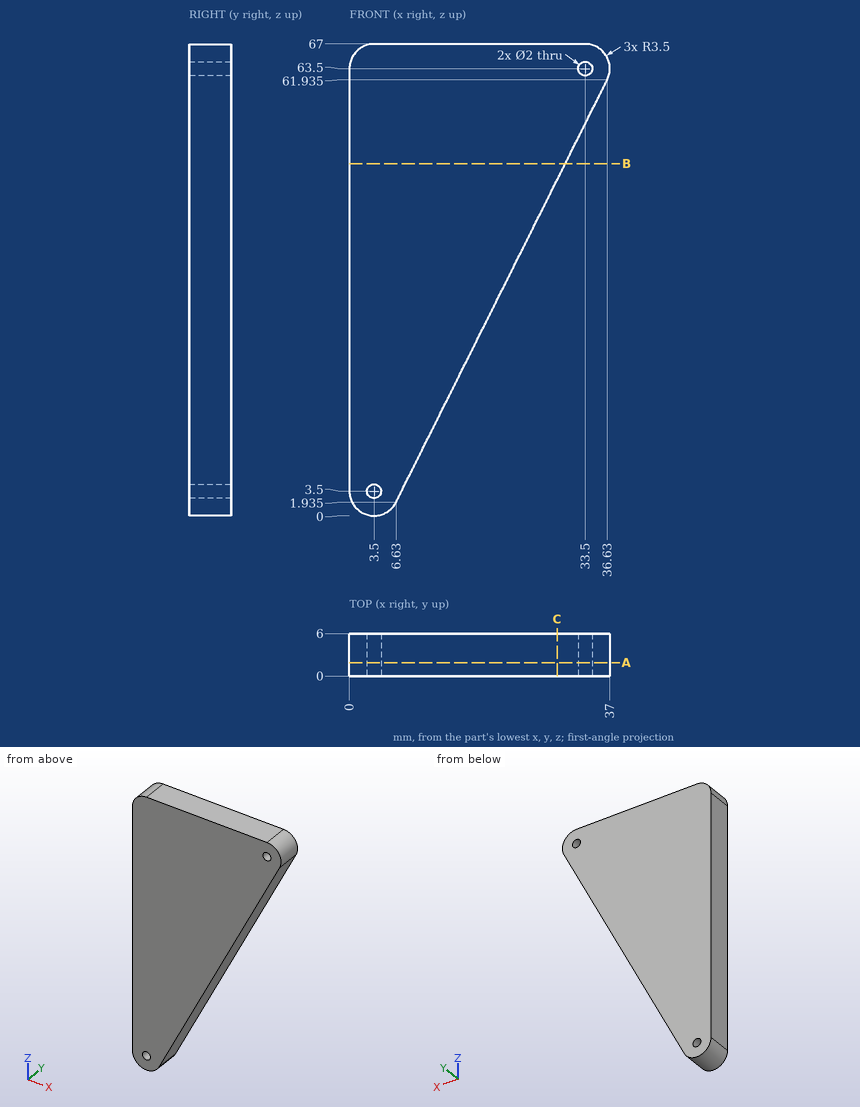
Answer from the drawing. Dimensions are ordinates in mm from the lowest x, y and z of the part. Give positions to 0.01 mm unless a question says otherwise; leave off trailing zeros. Write each loop counter-clockwise with the first axis right and the second up, starting at its lowest first coordinate (ties: lowest second). Pieces come first, ordered by that corner, then holes.
1) Section B-B (z = 50) is taken. Write down the section's boundary in (x, y), and give its area (3 significant figures).
2) Given P1, Ø3, axis at y = 2.5, z = 25.5, coming from the +X side, flat-ended and moving along its own axis, determine where the tip first touches the part or whether it passes through.
3) Find the intervals of material crossed by L1, parallel to X at y = 1.9, z = 63.5; L2, parallel to Z at x = 33.5, y = 4.75 (1 decimal); L3, parallel to X at y = 2.5, z = 3.5 (1 decimal), in increasing order.
4) Section C-C (x = 29.5) is taken. Write down the section's boundary in (y, z).
5) Section A-A (y = 1.9) is taken. Write down the section's boundary in (x, z) (1 decimal), and give its area (3 significant figures).
Response:
1. outline: (0, 0) - (30.66, 0) - (30.66, 6) - (0, 6) - close
1. area: 184 mm2
2. P1: stops at x = 19.16
3. L1: x = 0 to 32.5, 34.5 to 37
3. L2: z = 55.7 to 62.5, 64.5 to 67
3. L3: x = 0 to 2.5, 4.5 to 7.4
4. outline: (0, 47.67) - (6, 47.67) - (6, 67) - (0, 67) - close
5. outline: (0, 3.5) arc R3.5 ccw to (6.6, 1.9) - (36.6, 61.9) arc R3.5 ccw to (33.5, 67) - (3.5, 67) arc R3.5 ccw to (0, 63.5) - close; hole circle Ø2 at (3.5, 3.5); hole circle Ø2 at (33.5, 63.5)
5. area: 1,480 mm2
